from build123d import *

# Parameters (mm, degrees)
F0_R         = 19.05
F0_R_2       = 12.7
F2_DEPTH     = 69.85
F3_W         = 31.75
F3_H         = 127
F4_DEPTH     = 3.175
F5_R         = 12.7
F6_DEPTH     = 101.6
F7_R         = 12.7
F8_DEPTH     = 3.175
F9_R         = 12.7
F10_DEPTH    = 101.6
F6_FACE_R    = 19.05
F6_FACE_R_2  = 12.7
F13_REACH    = 74.5272199335
F10_FACE_R   = 19.05
F10_FACE_R_2 = 12.7
F14_REACH    = 74.5272199335


with BuildPart() as f2:
    # F0 (on Right) → F2 (new body, symmetric)
    with BuildSketch(Plane.YZ):
        Circle(F0_R)
        Circle(F0_R_2, mode=Mode.SUBTRACT)
    extrude(amount=F2_DEPTH, both=True)

    # F3 (on face) → F4 (join)
    with BuildSketch(Plane.YZ.offset(69.85)):
        with Locations((0, 44.45)):
            Rectangle(F3_W, F3_H)
    extrude(amount=F4_DEPTH)

    # F5 (on face) → F6 (join)
    with BuildSketch(Plane.YZ.offset(73.025)):
        with BuildLine():
            Line((15.875, 78.3697162906), (15.875, 99.4302837094))
            ThreePointArc((15.875, 99.4302837094), (9.0083459795, 105.6854759454), (-4.82e-08, 107.95))
            ThreePointArc((-4.82e-08, 107.95), (-9.0083460219, 105.6854759226), (-15.875, 99.4302837094))
            Line((-15.875, 99.4302837094), (-15.875, 78.3697162906))
            ThreePointArc((-15.875, 78.3697162906), (0, 69.85), (15.875, 78.3697162906))
        make_face()
        with Locations((0, 88.9)):
            Circle(F5_R, mode=Mode.SUBTRACT)
        with BuildLine():
            ThreePointArc((-15.875, 99.4302837094), (-19.05, 88.9), (-15.875, 78.3697162906))
            Line((-15.875, 78.3697162906), (-15.875, 99.4302837094))
        make_face()
        with BuildLine():
            ThreePointArc((15.875, 78.3697162906), (18.2389864028, 83.400738686), (19.05, 88.9))
            ThreePointArc((19.05, 88.9), (18.2389864028, 94.399261314), (15.875, 99.4302837094))
            Line((15.875, 99.4302837094), (15.875, 78.3697162906))
        make_face()
    extrude(amount=F6_DEPTH)

    # F7 (on face) → F8 (join)
    with BuildSketch(Plane(origin=(-69.85, 0, 0), x_dir=(0, -1, 0), z_dir=(-1, 0, 0))):
        with BuildLine():
            ThreePointArc((-15.875, 10.5302837094), (0, 19.05), (15.875, 10.5302837094))
            Line((15.875, 10.5302837094), (15.875, 107.95))
            Line((15.875, 107.95), (-15.875, 107.95))
            Line((-15.875, 107.95), (-15.875, 10.5302837094))
        make_face()
        with BuildLine():
            ThreePointArc((-15.875, -10.5302837094), (-9.0083460007, -16.785475934), (0, -19.05))
            ThreePointArc((0, -19.05), (9.0083460007, -16.785475934), (15.875, -10.5302837094))
            Line((15.875, -10.5302837094), (15.875, 10.5302837094))
            ThreePointArc((15.875, 10.5302837094), (0, 19.05), (-15.875, 10.5302837094))
            Line((-15.875, 10.5302837094), (-15.875, -10.5302837094))
        make_face()
        Circle(F7_R, mode=Mode.SUBTRACT)
        Circle(F7_R)
        with BuildLine():
            Line((0, -19.05), (15.875, -19.05))
            Line((15.875, -19.05), (15.875, -10.5302837094))
            ThreePointArc((15.875, -10.5302837094), (9.0083460007, -16.785475934), (0, -19.05))
        make_face()
        with BuildLine():
            Line((-15.875, -19.05), (0, -19.05))
            ThreePointArc((0, -19.05), (-9.0083460007, -16.785475934), (-15.875, -10.5302837094))
            Line((-15.875, -10.5302837094), (-15.875, -19.05))
        make_face()
    extrude(amount=F8_DEPTH)

    # F9 (on face) → F10 (join)
    with BuildSketch(Plane(origin=(-73.025, 0, 0), x_dir=(0, -1, 0), z_dir=(-1, 0, 0))):
        with BuildLine():
            Line((15.875, 78.3697162906), (15.875, 99.4302837094))
            ThreePointArc((15.875, 99.4302837094), (9.0083459795, 105.6854759454), (-4.82e-08, 107.95))
            ThreePointArc((-4.82e-08, 107.95), (-9.0083460219, 105.6854759226), (-15.875, 99.4302837094))
            Line((-15.875, 99.4302837094), (-15.875, 78.3697162906))
            ThreePointArc((-15.875, 78.3697162906), (0, 69.85), (15.875, 78.3697162906))
        make_face()
        with Locations((0, 88.9)):
            Circle(F9_R, mode=Mode.SUBTRACT)
        with BuildLine():
            ThreePointArc((15.875, 78.3697162906), (18.2389864028, 83.400738686), (19.05, 88.9))
            ThreePointArc((19.05, 88.9), (18.2389864028, 94.399261314), (15.875, 99.4302837094))
            Line((15.875, 99.4302837094), (15.875, 78.3697162906))
        make_face()
        with BuildLine():
            ThreePointArc((-15.875, 99.4302837094), (-19.05, 88.9), (-15.875, 78.3697162906))
            Line((-15.875, 78.3697162906), (-15.875, 99.4302837094))
        make_face()
    extrude(amount=F10_DEPTH)

    f13_end = Plane(origin=(153.9793167929, 0, 88.9), x_dir=(0.5, 0, -0.8660254038), z_dir=(-0.8660254038, 0, -0.5))
    # F6_face (on face) → F13 (cut, up to a plane its end follows)
    with BuildSketch(Plane(origin=(174.625, 0, 88.9), x_dir=(0, 1, 0), z_dir=(1, 0, 0))):
        Circle(F6_FACE_R)
        Circle(F6_FACE_R_2, mode=Mode.SUBTRACT)
    f13_long = extrude(amount=-F13_REACH, mode=Mode.PRIVATE)
    add(split(f13_long, bisect_by=f13_end, keep=Keep.BOTTOM, mode=Mode.PRIVATE), mode=Mode.SUBTRACT)

    f14_end = Plane(origin=(-153.9793167929, 0, 88.9), x_dir=(-0.5, 0, -0.8660254038), z_dir=(-0.8660254038, 0, 0.5))
    # F10_face (on face) → F14 (cut, up to a plane its end follows)
    with BuildSketch(Plane(origin=(-174.625, 0, 88.9), x_dir=(0, -1, 0), z_dir=(-1, 0, 0))):
        Circle(F10_FACE_R)
        Circle(F10_FACE_R_2, mode=Mode.SUBTRACT)
    f14_long = extrude(amount=-F14_REACH, mode=Mode.PRIVATE)
    add(split(f14_long, bisect_by=f14_end, keep=Keep.TOP, mode=Mode.PRIVATE), mode=Mode.SUBTRACT)


solid = f2.part
The model under review builds one solid part; all positions refer to its coordinate system, in mm. A direction names the side the tool comes from. Round coordinates to 2 decimals unless told otherwise and drop trailing zeros. Loops run counter-clockwise (first coordinate to the right, second up) from the corner with the lowest first, then second, coordinate; pieces in that order, holes last. Notation, with made-up numbers: M 16,-18 L 49,-18 A6 ccw 49,-7 Z; hole C 71.5,53 d4. An arc over 180 degrees is marked long. Answer as CSV lines item,"result".
1. Draft analysis for pull direction Y (two halves, no side actions). For faces 4 (the face through (69.85, -12, -17)), 5 (the face through (-116.637, -5.86, 77.633)), 6 (the face through (0.98, -15.12, -11.59)), state which applies: pulls with the +Y half, pulls with the -Y half, needs draft (parallel to the pull), parting line crosses it, or undercut.
Outcome:
face 4,"needs draft"
face 5,"undercut"
face 6,"parting line crosses it"
2. To check wall thickness, follow L1, parallel to X at y = 7, z = 86 (3 decimals); L2, parallel to X at y = 16, z = 89 (3 decimals); L3, parallel to Y at x = 121, z = 88.9. State the ranges of each line that lie inside material, in increasing order. Write a range as [from, to].
Outcome:
L1,"x = [-73.025, -69.85], [69.85, 73.025]"
L2,"x = [-153.922, -73.025], [73.025, 153.922]"
L3,"y = [-19.05, -12.7], [12.7, 19.05]"
3. We need section D-D (x = 51). Give the boundary of the cut face in (y, z), plus the area to 3 significant figures.
Outcome:
outline,"C 0,0 d38.1; hole C 0,0 d25.4"
area,"633 mm2"
4. We need section B-B (z = 25.5). Give the boundary of the cut face in (x, y) (3 decimals), plus the area to 3 significant figures.
Outcome:
outline,"M -73.025,-15.875 L -69.85,-15.875 L -69.85,15.875 L -73.025,15.875 Z; M 69.85,-15.875 L 73.025,-15.875 L 73.025,15.875 L 69.85,15.875 Z"
area,"202 mm2"
5. Insertion check: pin 1 Ø5 at (x, y) = (1.5, 10.5) entering from +Z; pin 2 Ø20.5 at (y, z) = (4.5, 0.5) entering from -X (3 decimals); pin 3 Ø2.5 at (y, z) = (9.5, 103.5) entering from +X. Each pin has a flat end and moves straight along its axis. Give the tip position at first contact, or say it passes through.
Outcome:
pin 1,"stops at z = 17.29"
pin 2,"stops at x = -73.025"
pin 3,"stops at x = 146.27"
6. We need section A-A (z = 0). Give the boundary of the cut face in (x, y) (3 decimals).
Outcome:
outline,"M -73.025,-15.875 L -69.85,-15.875 L -69.85,-19.05 L 69.85,-19.05 L 69.85,-15.875 L 73.025,-15.875 L 73.025,15.875 L 69.85,15.875 L 69.85,19.05 L -69.85,19.05 L -69.85,15.875 L -73.025,15.875 Z; hole M -69.85,-12.7 L 69.85,-12.7 L 69.85,12.7 L -69.85,12.7 Z"
7. For faces 1 (the face through (116.55, 5.86, 77.633)), 2 (the face through (73.025, 12, 105)), 3 (the face through (73.025, -12, 106)), list the 3-axis set-ups (+Z, -Z, +X, -X, +Y, -Y) from which the entire face can be reached by the end or side of a thin tool; tool diameter is ignored.
Outcome:
face 1,"+X"
face 2,"+Z, +X, +Y"
face 3,"+Z, +X, -Y"
